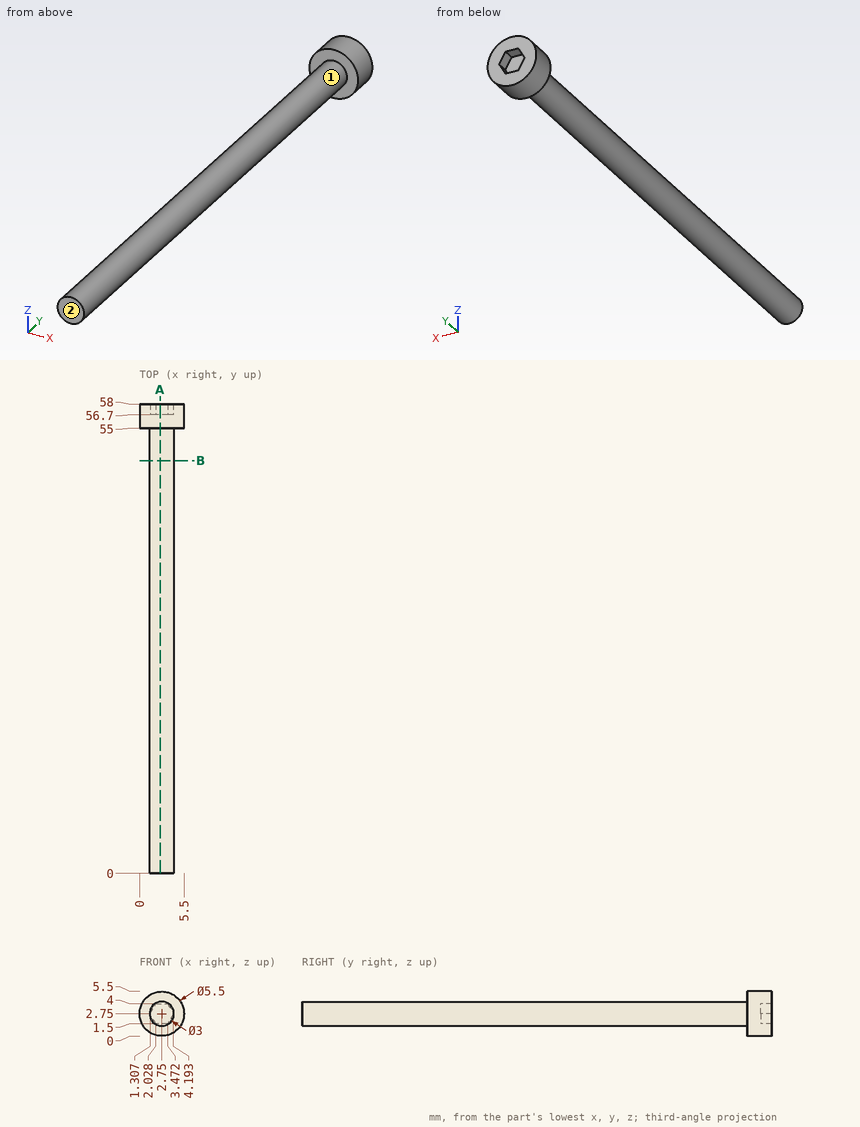
Print and shaded views of the part. All mm, measured from the part's lowest x, y and z. A direction names the side the tool comes from. Give positions to 0.01 mm unless a question says otherwise; leave off trailing zeros. Loops run counter-clockwise (first coordinate to the right, second up) from the corner with the lowest first, then second, coordinate; pieces in that order, holes last. Notation, with made-up numbers: (64.5, 79) - (95.5, 79) arc R12 ccw to (95.5, 84) - close; hole circle Ø5 at (23.5, 70.25). An arc over 180 degrees is marked (long way). Use a Markdown table: item, result.
(1) Wall check: line 1 along Y through (x, z) = (4.75, 1.55); line 2 along Z through (x, y) = (2.8, 3); line 3 along Y through (x, z) = (1.55, 2.7). Give the ranges that are in metal, low to high.
Taken from the geometry:
| item | result |
|---|---|
| line 1 | 55 to 58 |
| line 2 | 1.25 to 4.25 |
| line 3 | 0 to 56.7 |
(2) Which spindle directions (+Z, -Z, +X, -X, +Y, -Y) get a long thin tool onto all of the face, cutting with end or side? Do the marked faces 1 and 2. Say none if no direction does.
Taken from the geometry:
| item | result |
|---|---|
| face 1 | -Y |
| face 2 | +Z, -Z, +X, -X, -Y |
(3) Drop flat-ended pins along their axis: pin 1 Ø2 at (y, z) = (24, 4.5) entering from +X; pin 2 Ø1.5 at (y, z) = (17.5, 4.5) entering from -X. Give the stop position or say it passes through.
Taken from the geometry:
| item | result |
|---|---|
| pin 1 | x = 4.05 |
| pin 2 | x = 1.63 |
(4) Band-saw the part on B-B (y = 51). Give the cut face in (x, z).
Taken from the geometry:
| item | result |
|---|---|
| outline | circle Ø3 at (2.75, 2.75) |
(5) Band-saw the part on A-A (x = 2.55). Give the cut face in (y, z), and give its area (3 significant figures).
Taken from the geometry:
| item | result |
|---|---|
| outline | (0, 1.26) - (55, 1.26) - (55, 0.01) - (58, 0.01) - (58, 1.5) - (56.7, 1.5) - (56.7, 4) - (58, 4) - (58, 5.49) - (55, 5.49) - (55, 4.24) - (0, 4.24) - close |
| area | 177 mm2 |
